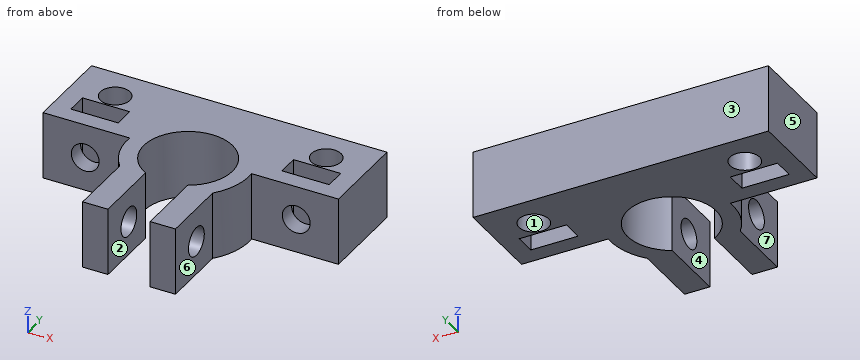
```python
from build123d import *

# Parameters (mm, degrees)
ESBO_O1_R                = 1.75
ESBO_O1_W                = 5.6
ESBO_O1_H                = 2.5
RESSALTO_EXTRUS_O1_DEPTH = 8
ESBO_O2_R                = 1.65
CORTE_EXTRUS_O1_DEPTH    = 7
ESBO_O3_R                = 1.7
CORTE_EXTRUS_O2_DEPTH    = 24


with BuildPart() as part:
    # Esboço1 → Ressalto-extrusão1 (new body)
    with BuildSketch(Plane.XY):
        with BuildLine():
            Line((17.5, 11), (0, 11))
            Line((0, 11), (-17.5, 11))
            Line((-17.5, 11), (-17.5, 0.55))
            Line((-17.5, 0.55), (-7.229107829, 0.55))
            ThreePointArc((-7.229107829, 0.55), (-6.889142873, -2.258807312), (-5.5, -4.723610907))
            Line((-5.5, -4.723610907), (-5.5, -12.723610907))
            Line((-5.5, -12.723610907), (-2.5, -12.723610907))
            Line((-2.5, -12.723610907), (-2.5, -4.616546328))
            ThreePointArc((-2.5, -4.616546328), (0, 5.25), (2.5, -4.616546328))
            Line((2.5, -4.616546328), (2.5, -12.723610907))
            Line((2.5, -12.723610907), (5.5, -12.723610907))
            Line((5.5, -12.723610907), (5.5, -4.723610907))
            ThreePointArc((5.5, -4.723610907), (6.889142873, -2.258807312), (7.229107829, 0.55))
            Line((7.229107829, 0.55), (17.5, 0.55))
            Line((17.5, 0.55), (17.5, 11))
        make_face()
        with Locations((12.5, 7)):
            Circle(ESBO_O1_R, mode=Mode.SUBTRACT)
        with Locations((-12.5, 7)):
            Circle(ESBO_O1_R, mode=Mode.SUBTRACT)
        with Locations((-12.5, 3.8)):
            Rectangle(ESBO_O1_W, ESBO_O1_H, mode=Mode.SUBTRACT)
        with Locations((12.5, 3.8)):
            Rectangle(ESBO_O1_W, ESBO_O1_H, mode=Mode.SUBTRACT)
    extrude(amount=RESSALTO_EXTRUS_O1_DEPTH)

    # Esboço2 → Corte-extrusão1 (cut)
    with BuildSketch(Plane.XZ.offset(-0.55)):
        with Locations((-12.5, 4)):
            Circle(ESBO_O2_R)
        with Locations((12.5, 4)):
            Circle(ESBO_O2_R)
    extrude(amount=-CORTE_EXTRUS_O1_DEPTH, mode=Mode.SUBTRACT)

    # Esboço3 → Corte-extrusão2 (cut, through all)
    with BuildSketch(Plane.ZY.offset(5.5)):
        with Locations((4, -8.223610907)):
            Circle(ESBO_O3_R)
    extrude(amount=-CORTE_EXTRUS_O2_DEPTH, mode=Mode.SUBTRACT)


solid = part.part
```
The model under review builds one solid part; all positions refer to its coordinate system, in mm. Face numbers are marked on the shaded views. A direction names the side the tool comes from. Round coordinates to 2 decimals unless told otherwise and drop trailing zeros. Write each loop counter-clockwise with the first axis right and the second up, starting at its lowest first coordinate (ties: lowest second). Pieces come first, ordered by that corner, then holes. Notation, with made-up numbers: M 2.5,-20 L 56.5,-20 A20 ccw 56.5,12 Z; hole C 31,66 d8. An arc over 180 degrees is marked long. Use CSV: the item, a comma, the result in double quotes. Start each with the question number.
(1) We need section A-A, the plane x = -12.5. State the section outline as (y, z) points.
(2) The part is to be moulded in two halves that separate along Y. For the marked faces 1, 2 and 3, say which applies: +Y half, -Y half, draft (parallel to the pull), parting line (faces both ways), or undercut.
(3) Tool access review of the marked faces 4, 5, 6 and 7: name each direction out of +Z, -Z, +X, -X, +Y, -Y from which nothing blocks a thin tool from reaching the whole face with its end or side.
(4) We need section C-C, the plane z = 1. State the section outline as (x, y) points.
(5) For line 1 along X through (y, z) = (5.75, 4); line 2 along X through (y, z) = (-6.5, 1.5); line 3 along Y through (x, z) = (13, 7), list the stretches that pass through material, from the lowest coordinate up.
(6) We need section B-B, the plane y = 0. State the section outline as (x, z) points.
(7) Clearance check with flat-ended pins moving along their axes: P1, Ø4.5, axis at x = -12.5, z = 4, coming from the -Y side; P2, Ø2, axis at x = -12.5, y = 7, coming from the -Z side. State where each tip first meets the part, or that it passes through.
(8) We need section D-D, the plane y = 7. State the section outline as (x, z) points, then the cut area to 3 significant figures.
Findings:
1,outline,"M 0.55,0 L 2.55,0 L 2.55,2.35 L 0.55,2.35 Z; M 0.55,5.65 L 2.55,5.65 L 2.55,8 L 0.55,8 Z; M 5.05,0 L 5.25,0 L 5.25,2.35 L 5.05,2.35 Z; M 5.05,5.65 L 5.25,5.65 L 5.25,8 L 5.05,8 Z; M 8.75,0 L 11,0 L 11,8 L 8.75,8 Z"
2,face 1,"undercut"
2,face 2,"draft"
2,face 3,"+Y half"
3,face 4,"+Z, -Z, -Y"
3,face 5,"+Z, -Z, -X, +Y, -Y"
3,face 6,"+Z, -Z, +X, -Y"
3,face 7,"+Z, -Z, -X, -Y"
4,outline,"M -17.5,0.55 L -7.23,0.55 A7.25 ccw -5.5,-4.72 L -5.5,-12.72 L -2.5,-12.72 L -2.5,-4.62 A5.25 cw long 2.5,-4.62 L 2.5,-12.72 L 5.5,-12.72 L 5.5,-4.72 A7.25 ccw 7.23,0.55 L 17.5,0.55 L 17.5,11 L -17.5,11 Z; hole M -15.3,2.55 L -9.7,2.55 L -9.7,5.05 L -15.3,5.05 Z; hole C -12.5,7 d3.5; hole M 9.7,2.55 L 15.3,2.55 L 15.3,5.05 L 9.7,5.05 Z; hole C 12.5,7 d3.5"
5,line 1,"-17.5 to -14.15, -10.85 to 10.85, 14.15 to 17.5"
5,line 2,"-5.5 to -2.5, 2.5 to 5.5"
5,line 3,"0.55 to 2.55, 5.05 to 5.32, 8.68 to 11"
6,outline,"M -7.25,0 L -5.25,0 L -5.25,8 L -7.25,8 Z; M 5.25,0 L 7.25,0 L 7.25,8 L 5.25,8 Z"
7,P1,"y = 0.55"
7,P2,"through"
8,outline,"M -17.5,0 L -14.25,0 L -14.25,8 L -17.5,8 Z; M -10.75,0 L 10.75,0 L 10.75,8 L -10.75,8 Z; M 14.25,0 L 17.5,0 L 17.5,8 L 14.25,8 Z"
8,area,"224 mm^2"
